The listing builds one solid part. Answer for the finished solid, in the listing's coordinates (mm). Face numbers are marked on the shaded views. A direction names the side the tool comes from. Round coordinates to 2 decimals unless told otherwise and drop trailing zeros. Order: outer loops, then holes, each group sorted by start corner. A loop starts at its lowest first (then second) coordinate and runs counter-clockwise, first axis right, second up. Notation, with made-up numbers: (-24.75, 74) -> (-19.75, 74) arc R20 cw to (-19.75, 91) -> close; hole circle Ø2 at (-24.75, 67). An arc over 180 degrees is marked (long way). Return JSON: item names as keys, results as strings. Group by question number.
(1) Determine the mould class of the marked faces 3, 4 and 5 for opening direction Y: +Y half, -Y half, draft (parallel to the pull), parting line (faces both ways), or undercut.
(2) The part is cut by section B-B (y = 15.24). Determine the outline of the cut face in (x, z).
(3) The part is cut by section A-A (x = 21). Determine the outline of the cut face in (y, z), plus the area to 3 significant figures.
(4) Which of the six approach directions +Z, -Z, +X, -X, +Y, -Y give full straight-line access (tool end or side, diameter ignored) to the marked faces 1 and 2?
(5) The part is cut by section D-D (z = 31.47). Determine the outline of the cut face in (x, y).
(6) Consider line 1 (Z direction, x = 17.78, y = 22.75); line 2 (X direction, y = 23.1, z = 31.47); line 3 (Y direction, x = 1.5, z = 5). Determine where each line is inside the solid, lowest interval first. Write a range as [from, to].
(7) The part is cut by section C-C (x = 15). Determine the outline of the cut face in (y, z).
(8) Each of these flat-tipped pins is pushed along its axis until it touches: pin 1 (5 mm diameter, centred on y = 7, z = 11, fed in from +X); pin 2 (12 mm diameter, centred on y = 2.5, z = 11.5, fed in from +X); pin 3 (1.5 mm diameter, centred on y = 21, z = 25, fed in from +X); pin 4 (3 mm diameter, centred on y = 15.24, z = 5, fed in from -X). Where does it stop, or does it pass through?
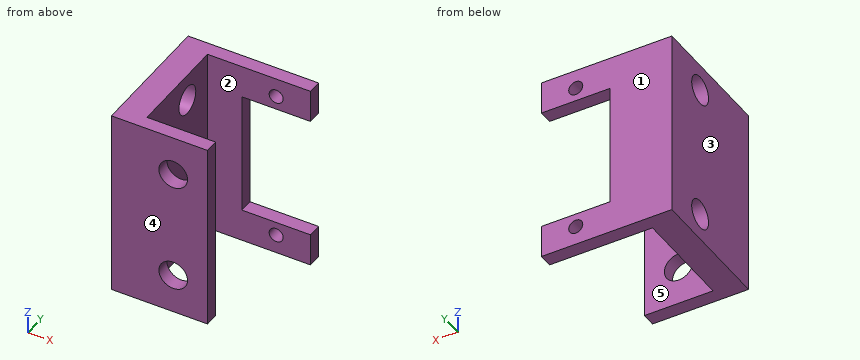
from build123d import *

# Parameters (mm, degrees)
SKETCH1_W                 = 5.08
SKETCH1_H                 = 19.05
BOSS_EXTRUDE1_DEPTH       = 35
F_5_0MM_DOWEL_HOLE1_D     = 5.3
F_5_0MM_DOWEL_HOLE2_D     = 5.3
F_5_0MM_DOWEL_HOLE2_DEPTH = 2.54
CUT_EXTRUDE1_REACH        = 50.883
SKETCH6_W                 = 12.7
SKETCH6_H                 = 22.86
M2_CLEARANCE_HOLE1_D      = 2.6
M2_CLEARANCE_HOLE1_DEPTH  = 2.54


with BuildPart() as part:
    # Sketch1 → Boss-Extrude1 (new body)
    with BuildSketch(Plane.XY):
        Polygon((0, 2.54), (0, 0), (17.78, 0), (17.78, 2.54), (5.08, 2.54), align=None)
        with Locations((2.54, 12.065)):
            Rectangle(SKETCH1_W, SKETCH1_H)
        Polygon((0, 24.13), (0, 21.59), (5.08, 21.59), (24.13, 21.59), (24.13, 24.13), align=None)
    extrude(amount=BOSS_EXTRUDE1_DEPTH)

    # Ø5.0mm Dowel Hole1 (through all)
    with Locations(Plane(origin=(5.08, 0, 0), x_dir=(0, 0, -1), z_dir=(1, 0, 0))):
        with Locations((-30, 15.24), (-5, 15.24)):
            Hole(F_5_0MM_DOWEL_HOLE1_D / 2)

    # Ø5.0mm Dowel Hole2
    with Locations(Plane(origin=(0, 2.54, 0), x_dir=(1, 0, 0), z_dir=(0, 1, 0))):
        with Locations((11.43, -27.66), (11.43, -7.34)):
            Hole(F_5_0MM_DOWEL_HOLE2_D / 2, depth=F_5_0MM_DOWEL_HOLE2_DEPTH)

    # Sketch6 → Cut-Extrude1 (cut, up to next)
    with BuildSketch(Plane(origin=(0, 24.13, 0), x_dir=(1, 0, 0), z_dir=(0, 1, 0)), mode=Mode.PRIVATE) as cut_extrude1_sk1:
        with Locations((17.78, -17.5)):
            Rectangle(SKETCH6_W, SKETCH6_H)
    cut_extrude1_tool1 = extrude(cut_extrude1_sk1.sketch, amount=-CUT_EXTRUDE1_REACH, mode=Mode.PRIVATE) & part.part
    add(cut_extrude1_tool1.solids().sort_by_distance((17.78, 24.13, 17.5))[0], mode=Mode.SUBTRACT)

    # M2 Clearance Hole1
    with Locations(Plane(origin=(0, 24.13, 0), x_dir=(1, 0, 0), z_dir=(0, 1, 0))):
        with Locations((17.78, -31.47), (17.78, -3.53)):
            Hole(M2_CLEARANCE_HOLE1_D / 2, depth=M2_CLEARANCE_HOLE1_DEPTH)


solid = part.part
Answer below:
{
 "1": {"face 3": "draft", "face 4": "-Y half", "face 5": "undercut"},
 "2": {"outline": "(0, 0) -> (5.08, 0) -> (5.08, 2.35) -> (0, 2.35) -> close; (0, 7.65) -> (5.08, 7.65) -> (5.08, 27.35) -> (0, 27.35) -> close; (0, 32.65) -> (5.08, 32.65) -> (5.08, 35) -> (0, 35) -> close"},
 "3": {"outline": "(21.59, 0) -> (24.13, 0) -> (24.13, 6.07) -> (21.59, 6.07) -> close; (21.59, 28.93) -> (24.13, 28.93) -> (24.13, 35) -> (21.59, 35) -> close", "area": "30.8 mm²"},
 "4": {"face 1": "+Z, -Z, +X, -X, +Y", "face 2": "+Z, -Z, +X"},
 "5": {"outline": "(0, 0) -> (17.78, 0) -> (17.78, 2.54) -> (5.08, 2.54) -> (5.08, 13.04) -> (0, 13.04) -> close; (0, 17.44) -> (5.08, 17.44) -> (5.08, 21.59) -> (16.48, 21.59) -> (16.48, 24.13) -> (0, 24.13) -> close; (19.08, 21.59) -> (24.13, 21.59) -> (24.13, 24.13) -> (19.08, 24.13) -> close"},
 "6": {"line 1": "z = [0, 2.23], [4.83, 6.07], [28.93, 30.17], [32.77, 35]", "line 2": "x = [0, 16.48], [19.08, 24.13]", "line 3": "y = [0, 12.59], [17.89, 24.13]"},
 "7": {"outline": "(0, 0) -> (2.54, 0) -> (2.54, 35) -> (0, 35) -> close; (21.59, 0) -> (24.13, 0) -> (24.13, 6.07) -> (21.59, 6.07) -> close; (21.59, 28.93) -> (24.13, 28.93) -> (24.13, 35) -> (21.59, 35) -> close"},
 "8": {"pin 1": "stops at x = 5.08", "pin 2": "stops at x = 17.78", "pin 3": "stops at x = 11.43", "pin 4": "passes through"}
}
